Can you work these out from the model? Positions are in its coordinate system, mm. A direction names the side the tool comes from. Coordinates: 2 decimals unless noted, no trailing zeros. Write each loop counter-clockwise with the first axis right and the second up, starting at its lowest first coordinate (ties: lowest second). Pieces come first, ordered by that corner, then holes. Notation, with made-up numbers: (40, 57) -> (47, 57) arc R31 cw to (47, 87) -> close; hole circle Ø2 at (-38.5, -1). An arc over 180 degrees is marked (long way). Answer as CSV lines item,"result". Start each with the question number.
```python
from build123d import *

# Parameters (mm, degrees)
F0_R     = 69
F0_R_2   = 3.25
F1_DEPTH = 8
F2_R     = 19.45
F2_R_2   = 12.5
F3_DEPTH = 10
F4_R     = 3


with BuildPart() as f1:
    # F0 (on Top) → F1 (new body)
    with BuildSketch(Plane.XY):
        Circle(F0_R)
        with Locations((0, -63)):
            Circle(F0_R_2, mode=Mode.SUBTRACT)
        with Locations((-63, 0)):
            Circle(F0_R_2, mode=Mode.SUBTRACT)
        with Locations((63, 0)):
            Circle(F0_R_2, mode=Mode.SUBTRACT)
        with Locations((0, 63)):
            Circle(F0_R_2, mode=Mode.SUBTRACT)
    extrude(amount=F1_DEPTH)

    # F2 (on face) → F3 (join)
    with BuildSketch(Plane.XY.offset(8)):
        Circle(F2_R)
        Circle(F2_R_2, mode=Mode.SUBTRACT)
    extrude(amount=F3_DEPTH)

    # F4
    f4_edges = [f1.edges().sort_by_distance(p)[0] for p in [
        (-12.5, 0, 8),
    ]]
    fillet(f4_edges, radius=F4_R)


solid = f1.part
```
Q1. Which directions (+Z, -Z, +X, -X, +Y, -Y) give clear straight access to the entire face, cutting with the end or side of a thin tool? Please do faces 4 (the face through (-15.43, -11.84, 12.93)), 5 (the face through (0, -13, 18)).
Q2. Imagine slicing it at A-A (x = 0). Write out the boundary of the cut face in (y, z).
Q3. If we mould it in two halves opening along Y, with no side actions, what happens to faces 1 (the face through (-1, 1, 0)), 2 (the face through (-2.395, 65.197, 3.944)), 3 (the face through (65.814, 20.726, 3.944))? For each: released by +Y, released by -Y, zero draft, split by the parting line, or undercut.
Q4. Imagine slicing it at C-C (x = 63). Write out the boundary of the cut face in (y, z), then the cut area to 3 significant figures.
Q5. For pin 1 (5 mm diameter, centred on x = -4, y = -26, fed in from +Z); pin 2 (10 mm diameter, centred on x = -6.5, y = -2, fed in from +Z); pin 3 (5 mm diameter, centred on y = 49.5, z = 4, fed in from +X), each with a flat end and sliding along its axis, tell me the tip position at first contact or that it passes through.
Q6. I need wall thicknesses on L1, parallel to Y at x = 0, z = 4.25; L2, parallel to Z at x = 45, y = -50.5; L3, parallel to X at y = 3, z = 14. Which ranges of each line are inside material? Lowest first, please.
Q7. Imagine slicing it at D-D (z = 13). Write out the boundary of the cut face in (x, y), then the cut area to 3 significant figures.
Entries:
1,face 4,"+Z"
1,face 5,"+Z, +X, -X, +Y, -Y"
2,outline,"(-69, 0) -> (-66.25, 0) -> (-66.25, 8) -> (-69, 8) -> close; (-59.75, 0) -> (59.75, 0) -> (59.75, 8) -> (19.45, 8) -> (19.45, 18) -> (12.5, 18) -> (12.5, 11) arc R3 cw to (9.5, 8) -> (-9.5, 8) arc R3 cw to (-12.5, 11) -> (-12.5, 18) -> (-19.45, 18) -> (-19.45, 8) -> (-59.75, 8) -> close; (66.25, 0) -> (69, 0) -> (69, 8) -> (66.25, 8) -> close"
3,face 1,"zero draft"
3,face 2,"undercut"
3,face 3,"split by the parting line"
4,outline,"(-28.14, 0) -> (-3.25, 0) -> (-3.25, 8) -> (-28.14, 8) -> close; (3.25, 0) -> (28.14, 0) -> (28.14, 8) -> (3.25, 8) -> close"
4,area,"398 mm2"
5,pin 1,"z = 8"
5,pin 2,"z = 9.07"
5,pin 3,"x = 50.52"
6,L1,"-69 to -66.25, -59.75 to 59.75, 66.25 to 69"
6,L2,"0 to 8"
6,L3,"-19.22 to -12.13, 12.13 to 19.22"
7,outline,"circle Ø38.9 at (0, 0); hole circle Ø25 at (0, 0)"
7,area,"698 mm2"
